from build123d import *

# Parameters (mm, degrees)
BOSS_EXTRUDE1_DEPTH = 12.7
SKETCH2_R           = 1.0033
CUT_EXTRUDE1_DEPTH  = 66.979539467
FILLET1_R           = 7.62


with BuildPart() as part:
    # Sketch1 → Boss-Extrude1 (new body)
    with BuildSketch(Plane(origin=(0, 0, 0), x_dir=(1, 0, 0), z_dir=(0, 1, 0))):
        with BuildLine():
            ThreePointArc((12.7, -62.217039467), (0, -63.5), (-12.7, -62.217039467))
            Line((-12.7, -62.217039467), (-12.7, -66.979539467))
            Line((-12.7, -66.979539467), (12.7, -66.979539467))
            Line((12.7, -66.979539467), (12.7, -62.217039467))
        make_face()
    extrude(amount=BOSS_EXTRUDE1_DEPTH)

    # Sketch2 → Cut-Extrude1 (cut)
    with BuildSketch(Plane.XY):
        with Locations(Location((-5.644444444, 6.35, 0), (0, 0, 180))):
            Circle(SKETCH2_R)
    cut_extrude1 = extrude(amount=CUT_EXTRUDE1_DEPTH, mode=Mode.SUBTRACT)

    # Mirror1: Cut-Extrude1 across plane
    add(cut_extrude1.mirror(Plane(origin=(0, 0, 0), x_dir=(0, 0, 1), z_dir=(1, 0, 0))), mode=Mode.SUBTRACT)

    # Fillet1
    fillet1_edges = [part.edges().sort_by_distance(p)[0] for p in [
        (12.7, 0, 64.598289467),
        (-12.7, 0, 64.598289467),
    ]]
    fillet(fillet1_edges, radius=FILLET1_R)


solid = part.part
Check sheet for the modelled part. Datum: model origin and axes. Units: mm. Round coordinates to 2 decimals unless told otherwise and drop trailing zeros. Write each loop counter-clockwise with the first axis right and the second up, starting at its lowest first coordinate (ties: lowest second). Pieces come first, ordered by that corner, then holes. Notation, with made-up numbers: (17.25, -14) -> (68.25, -14) arc R10 cw to (68.25, -9) -> close; hole circle Ø5 at (-37, 78.25). An arc over 180 degrees is marked (long way). Answer as CSV lines item,"result". Start each with the question number.
1) Release check for a two-part mould opening along Y. For faces 1 (the flat face through (0, 12.7, 65)), 2 (the cylindrical face through (6.18, 5.5, 65.04)), 3 (the flat face through (0, 6, 66.98)) record: pulls with the +Y half, pulls with the -Y half, needs draft (parallel to the pull), parting line crosses it, or undercut.
2) Material ranges on line 1 (X direction, y = 6, z = 65.7); line 2 (X direction, y = 6.35, z = 65.75); line 3 (Z direction, x = 0.5, y = 0.5), recorded low to high. Write a range as from..to.
3) Go/stop test with flat-tipped pins: P1, Ø3, axis at x = 1, y = 6, coming from the -Z side; P2, Ø2.5, axis at x = 5.64, y = 6.35, coming from the -Z side; P3, Ø1.5, axis at y = 5.5, z = 66.5, coming from the +X side. Record where each tip stops, or that it passes through.
4) Section check D-D on x = 8.5. Enter the section's corners in (y, z), and give its area (3 significant figures).
5) Section check A-A on z = 64.35. Enter the section's corners in (x, y).
6) Section check C-C on y = 10. Enter the section's corners in (x, z).
7) Section check B-B on y = 6.35. Enter the section's corners in (x, z), and give its area (3 significant figures).
Found:
1,face 1,"pulls with the +Y half"
1,face 2,"undercut"
1,face 3,"needs draft"
2,line 1,"x = -12.53..-6.58, -4.7..4.7, 6.58..12.53"
2,line 2,"x = -12.59..-6.65, -4.64..4.64, 6.65..12.59"
2,line 3,"z = 63.5..66.98"
3,P1,"stops at z = 63.45"
3,P2,"stops at z = 63.13"
3,P3,"stops at x = 12.58"
4,outline,"(0.81, 62.93) -> (12.7, 62.93) -> (12.7, 66.98) -> (0.81, 66.98) -> close"
4,area,"48.2 mm^2"
5,outline,"(-12.7, 7.62) arc R7.62 ccw to (-5.08, 0) -> (5.08, 0) arc R7.62 ccw to (12.7, 7.62) -> (12.7, 12.7) -> (-12.7, 12.7) -> close; hole circle Ø2.01 at (-5.64, 6.35); hole circle Ø2.01 at (5.64, 6.35)"
6,outline,"(-12.7, 62.22) arc R63.5 cw to (12.7, 62.22) -> (12.7, 66.98) -> (-12.7, 66.98) -> close"
7,outline,"(-12.59, 62.24) arc R63.5 cw to (-6.65, 63.15) -> (-6.65, 66.98) -> (-12.59, 66.98) -> close; (-4.64, 63.33) arc R63.5 cw to (4.64, 63.33) -> (4.64, 66.98) -> (-4.64, 66.98) -> close; (6.65, 63.15) arc R63.5 cw to (12.59, 62.24) -> (12.59, 66.98) -> (6.65, 66.98) -> close"
7,area,"83.2 mm^2"
